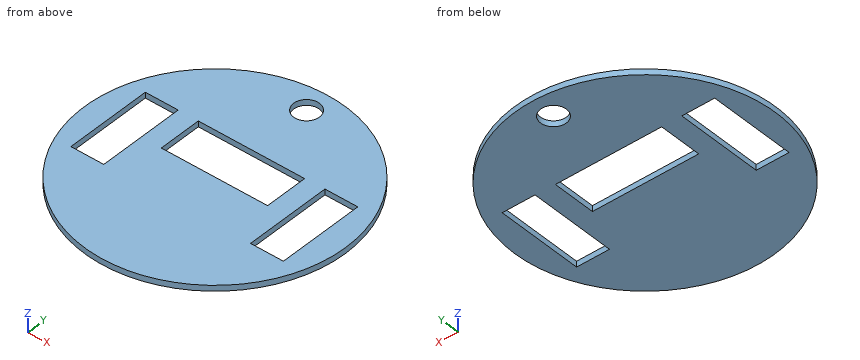
from build123d import *

# Parameters (mm, degrees)
SKETCH1_R           = 312.497780416
SKETCH1_R_2         = 30.815082176
SKETCH1_W           = 78.780158854
SKETCH1_H           = 207.033394325
SKETCH1_H_2         = 207.033394324
SKETCH1_W_2         = 254.787899309
SKETCH1_H_3         = 103.031623715
BOSS_EXTRUDE1_DEPTH = 13.716


with BuildPart() as part:
    # Sketch1 → Boss-Extrude1 (new body)
    with BuildSketch(Plane.XY):
        Circle(SKETCH1_R)
        with Locations((0, 254.843469114)):
            Circle(SKETCH1_R_2, mode=Mode.SUBTRACT)
        with Locations((213.217227107, 0.764216519)):
            Rectangle(SKETCH1_W, SKETCH1_H, mode=Mode.SUBTRACT)
        with Locations((-216.277951012, -0.485073447)):
            Rectangle(SKETCH1_W, SKETCH1_H_2, mode=Mode.SUBTRACT)
        with Locations((-1.212629894, 51.515811858)):
            Rectangle(SKETCH1_W_2, SKETCH1_H_3, mode=Mode.SUBTRACT)
    extrude(amount=BOSS_EXTRUDE1_DEPTH)


solid = part.part
Check sheet for the modelled part. Datum: model origin and axes. Units: mm. Round coordinates to 2 decimals unless told otherwise and drop trailing zeros. Order: outer loops, then holes, each group sorted by start corner. A loop starts at its lowest first (then second) coordinate and runs counter-clockwise, first axis right, second up.
Q1. Cross-section at C-C, the plane x = 228.5. Enter the section's corners in (y, z), plus the area to 3 significant figures.
Filled sheet:
outline: (-213.17, 0) - (-102.75, 0) - (-102.75, 13.72) - (-213.17, 13.72) - close; (104.28, 0) - (213.17, 0) - (213.17, 13.72) - (104.28, 13.72) - close
area: 3,010 mm2
Q2. Cross-section at D-D, the plane y = 89. Enter the section's corners in (x, z).
Filled sheet:
outline: (-299.56, 0) - (-255.67, 0) - (-255.67, 13.72) - (-299.56, 13.72) - close; (-176.89, 0) - (-128.61, 0) - (-128.61, 13.72) - (-176.89, 13.72) - close; (126.18, 0) - (173.83, 0) - (173.83, 13.72) - (126.18, 13.72) - close; (252.61, 0) - (299.56, 0) - (299.56, 13.72) - (252.61, 13.72) - close
Q3. Scan lines: L1, parallel to Y at x = 0, z = 11.25; L2, parallel to Y at x = -2, z = 6; L3, parallel to X at y = -67, z = 9.25. Record each from-to range of solid material in increasing order.
Filled sheet:
L1: y = -312.5 to 0, 103.03 to 224.03, 285.66 to 312.5
L2: y = -312.49 to 0, 103.03 to 224.09, 285.59 to 312.49
L3: x = -305.23 to -255.67, -176.89 to 173.83, 252.61 to 305.23
Q4. Cross-section at A-A, the plane x = 0. Enter the section's corners in (y, z).
Filled sheet:
outline: (-312.5, 0) - (0, 0) - (0, 13.72) - (-312.5, 13.72) - close; (103.03, 0) - (224.03, 0) - (224.03, 13.72) - (103.03, 13.72) - close; (285.66, 0) - (312.5, 0) - (312.5, 13.72) - (285.66, 13.72) - close
Q5. Cross-section at B-B, the plane y = -44. Enter the section's corners in (x, z), plus the area to 3 significant figures.
Filled sheet:
outline: (-309.38, 0) - (-255.67, 0) - (-255.67, 13.72) - (-309.38, 13.72) - close; (-176.89, 0) - (173.83, 0) - (173.83, 13.72) - (-176.89, 13.72) - close; (252.61, 0) - (309.38, 0) - (309.38, 13.72) - (252.61, 13.72) - close
area: 6,330 mm2
Q6. Depth check by flat-ended pin: P1, Ø1.5, axis at x = 117.5, z = 3, coming from the +Y side; P2, Ø4, axis at x = -51.5, z = 5, coming from the +Y side; P3, Ø7, axis at y = 64, z = 9.5, coming from the +X side; P4, Ø6, axis at x = -15.5, y = 204, coming from the -Z side. Enter the tip coordinate at first touch or a pass-through.
Filled sheet:
P1: stops at y = 289.87
P2: stops at y = 308.55
P3: stops at x = 306.59
P4: stops at z = 0
